Build history of the part. All positions in model axes, mm. A direction names the side the tool comes from. Round coordinates to 2 decimals unless told otherwise and drop trailing zeros. Write each loop counter-clockwise with the first axis right and the second up, starting at its lowest first coordinate (ties: lowest second). Pieces come first, ordered by that corner, then holes. Notation, with made-up numbers: M -35.75,40.25 L 18.25,40.25 A19 cw 18.25,66.25 Z; hole C 37.5,53 d9. An arc over 180 degrees is marked long. Write item = value, one per line. Start each with the question number.
Q1. Band-saw the part on B-B on y = -60. Write the cut outline in (x, z), plus the area to 3 significant figures.
Q2. Tool access for faces 1 (the flat face through (40.9, -58.7, 3.6)), 2 (the flat face through (-16.12, -21.46, 3.63)): list every direction of +Z, -Z, +X, -X, +Y, -Y with a clear straight run to the whole face (end or side of a thin tool).
Q3. Band-saw the part on A-A on z = 3.25. Write the cut outline in (x, y), plus the area to 3 significant figures.
Q4. Probe L1, parallel to Y at x = 19, z = 2.5; L2, parallel to X at y = -9, z = 1.5; L3, parallel to Y at x = 26, z = 4.5. List the from-to ranges inside material, lowest first.
Q5. Band-saw the part on C-C on x = 39.5. Write the cut outline in (y, z).
Q6. Pull direction X, two halves, no side cores. Call faces 3 (the flat face through (26.76, -55.6, 3.63)), 4 (the flat face through (-4.657, -5.702, 3.631)), 5 (the flat face through (25, -26, 7.366)): released by +X, released by -X, zero draft, split by the parting line, or undercut.
Q7. Band-saw the part on D-D on y = -12. Write the cut outline in (x, z).
Q8. Drop flat-ended pins along their axis: P1, Ø1.5, axis at x = 14, z = 2, coming from the +Y side; P2, Ø1.5, axis at x = 25.5, z = 5, coming from the +Y side. Give the stop position or say it passes through.
```python
from build123d import *

# Parameters (mm, degrees)
F1_DEPTH = 7.366


with BuildPart() as f1:
    # F0 (on Top) → F1 (new body)
    with BuildSketch(Plane.XY):
        Polygon((15.7023970503, -0.3485125312), (14.3449331899, 0.5018823129), (0.7010700917, -4.2930147397), align=None)
        Polygon((72.1815829965, 14.5023252855), (15.7023970503, -0.3485125312), (37.6951557319, -14.1260642838), (40.8171921849, -41.502378915), (32.3127703641, -50.0298144352), (49.7593244376, -67.6403014412), align=None)
        Polygon((37.6951557319, -14.1260642838), (15.7023970503, -0.3485125312), (0.7010700917, -4.2930147397), (-9.4604333978, -7.8640974148), (32.3127703641, -50.0298144352), (40.8171921849, -41.502378915), align=None)
        Polygon((-9.4604333978, -7.8640974148), (0.7010700917, -4.2930147397), (-10.1671477618, -7.1507425556), align=None)
        Polygon((32.3127703641, -50.0298144352), (-9.4604333978, -7.8640974148), (-11.6502816094, -8.633681268), (-20.7155617162, -34.6534893185), (-6.0245663122, -57.9640956692), (21.3600854217, -61.0121382883), align=None)
    extrude(amount=F1_DEPTH)


solid = f1.part
```
Conclusion:
q1.outline = M 12.27,0 L 22.37,0 L 22.37,7.37 L 12.27,7.37 Z; M 42.19,0 L 51.84,0 L 51.84,7.37 L 42.19,7.37 Z
q1.area = 146 mm^2
q2.face_1 = +Z, -Z, -Y
q2.face_2 = +Z, -Z, -X, +Y
q3.outline = M -20.72,-34.65 L -6.02,-57.96 L 21.36,-61.01 L 32.31,-50.03 L 49.76,-67.64 L 72.18,14.5 L 15.7,-0.35 L 14.34,0.5 L 0.7,-4.29 L -10.17,-7.15 L -9.46,-7.86 L -11.65,-8.63 Z
q3.area = 4,640 mm^2
q4.L1 = -60.75 to 0.52
q4.L2 = -11.78 to 65.77
q4.L3 = -56.36 to 2.36
q5.outline = M -57.28,0 L 5.91,0 L 5.91,7.37 L -57.28,7.37 Z
q6.face_3 = undercut
q6.face_4 = released by -X
q6.face_5 = zero draft
q7.outline = M -12.82,0 L 64.95,0 L 64.95,7.37 L -12.82,7.37 Z
q8.P1 = 0.5
q8.P2 = 2.42
